Autodesk Inventor part; units mm, degrees
ref_plane "YZ Plane" through (0, 0, 0) normal (1, 0, 0) x (0, 1, 0)
ref_plane "XZ Plane" through (0, 0, 0) normal (0, 1, 0) x (-1, 0, 0)
ref_plane "XY Plane" through (0, 0, 0) normal (0, 0, 1) x (1, 0, 0)
ref_plane "Work Plane1" through (0, 0, -290) normal (1, 0, 0) x (0, 1, 0)
sketch "Sketch1" plane through (0, 0, -290) normal (1, 0, 0) x (0, 1, 0)
  circle A0 centre (-627.5, 172.5) radius 11 construction
  circle A1 centre (-627.5, 172.5) radius 4 construction
  line L0 (-655, 150) -> (-605, 150)
  line L1 (-605, 150) -> (-605, 195)
  line L2 (-605, 195) -> (-655, 195)
  line L3 (-655, 195) -> (-655, 150)
  circle A2 centre (-627.5, 172.5) radius 16 construction
  line L4 (0, 0) -> (-700, 0)
  line L5 (-700, -55) -> (-700, 580)
  circle A3 centre (-627.5, 172.5) radius 4
  line L6 (-649.7, 155.3) -> (-610.3, 155.3)
  line L7 (-610.3, 155.3) -> (-610.3, 189.7)
  line L8 (-610.3, 189.7) -> (-649.7, 189.7)
  line L9 (-649.7, 189.7) -> (-649.7, 155.3)
  point P0 (0, 290)
  dimension "d0" = 22
  dimension "d1" = 8
  dimension "d2" = 45
  dimension "d3" = 50
  dimension "d4" = 5
  dimension "d7" = 22.5
  dimension "d8" = 22.5
  dimension "d10" = 5.3
  dimension "d13" = 150
  dimension "d14" = 95
extrude "Extrusion1" add sketch "Sketch1" along normal blind 3 contours L9 L8 L7 L6
properties part number "cord roller"
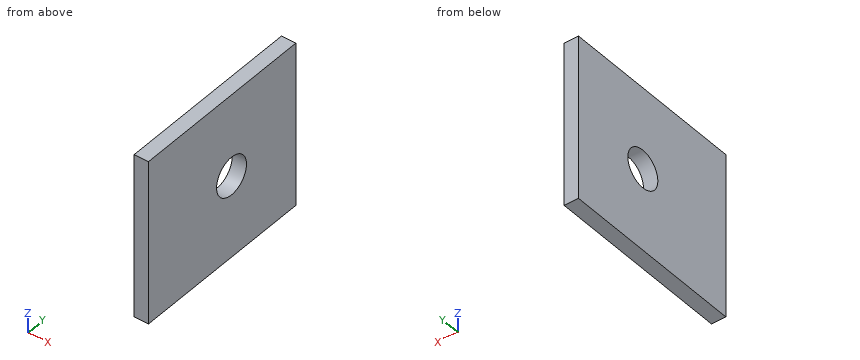
Input: part model. Units: mm. Frame: model coordinates. Give positions to 0.01 mm unless a question says otherwise; leave off trailing zeros. Order: outer loops, then holes, each group sorted by start corner. A loop starts at its lowest first (then second) coordinate and runs counter-clockwise, first axis right, second up. Notation, with made-up numbers: (-11, 3.25) - (46, 3.25) arc R29 ccw to (46, 25.25) - close; hole circle Ø1 at (87, 69). An arc over 180 degrees is marked (long way). Put each result on its own line as item: value.
Item 1: Section query A-A, the plane y = -627.5. Return loops of the section in (x, z), then the cut area to 3 significant figures.
Found:
outline: (0, -134.7) - (3, -134.7) - (3, -121.5) - (0, -121.5) - close; (0, -113.5) - (3, -113.5) - (3, -100.3) - (0, -100.3) - close
area: 79.2 mm^2
Item 2: Section query B-B, the plane z = -117.5. Return loops of the section in (x, y), then the cut area to 3 significant figures.
Found:
outline: (0, -649.7) - (3, -649.7) - (3, -631.5) - (0, -631.5) - close; (0, -623.5) - (3, -623.5) - (3, -610.3) - (0, -610.3) - close
area: 94.2 mm^2
Item 3: Section query C-C, the plane x = 0.7. Return loops of the section in (y, z).
Found:
outline: (-649.7, -134.7) - (-610.3, -134.7) - (-610.3, -100.3) - (-649.7, -100.3) - close; hole circle Ø8 at (-627.5, -117.5)
Item 4: Ray query, L1, parallel to Z at x = 2.45, y = -627.5. Return the intervals inside material, ascending. Write a range as from..to.
Found:
L1: z = -134.7..-121.5, -113.5..-100.3
